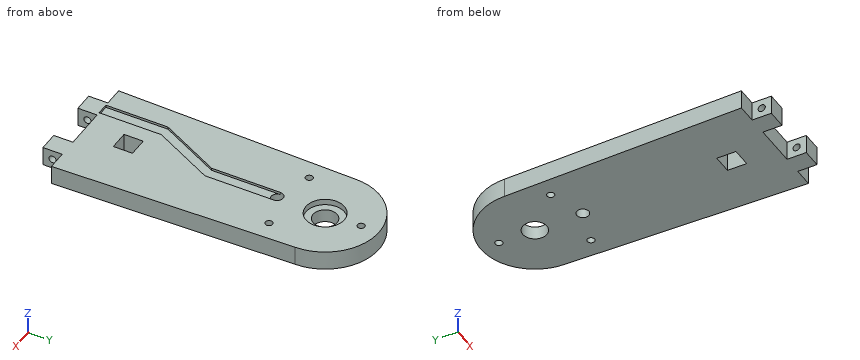
```python
from build123d import *

# Parameters (mm, degrees)
ARM_BOSS_EXTRUDE1_DEPTH                    = 8
SKETCH2_R                                  = 8
BEARING_CUT_EXTRUDE1_DEPTH                 = 2.5
SKETCH3_R                                  = 5
SHAFT_HOLE_CUT_EXTRUDE2_DEPTH              = 5.5
SKETCH4_R                                  = 2.5
CABLE_HOLE_CUT_EXTRUDE3_DEPTH              = 8
SKETCH5_W                                  = 8
SKETCH5_H                                  = 8
PUZZLE_SLOT_BOSS_EXTRUDE2_DEPTH            = 8
SKETCH6_W                                  = 5
SKETCH6_H                                  = 7.5
CABLE_CUT_EXTRUDE4_DEPTH                   = 1
SKETCH7_R                                  = 1.5
MOUNTING_HOLES_CUT_EXTRUDE5_DEPTH          = 8
PUZZLE_SLOT_SCREW_HOLES_CUT_EXTRUDE6_REACH = 118.155
SKETCH8_R                                  = 1.5
SIDE_PUZZLE_SLOT_CUT_EXTRUDE7_DEPTH        = 8
CABLE_LOWER_CUT_EXTRUDE8_DEPTH             = 1


with BuildPart() as part:
    # Sketch1 → Arm Boss-Extrude1 (new body)
    with BuildSketch(Plane.XY):
        with BuildLine():
            Line((-22.5, 0), (-25, -100))
            Line((-25, -100), (0, -100))
            Line((0, -100), (25, -100))
            Line((25, -100), (22.5, 0))
            ThreePointArc((22.5, 0), (0, 22.5), (-22.5, 0))
        make_face()
    extrude(amount=-ARM_BOSS_EXTRUDE1_DEPTH)

    # Sketch2 → Bearing Cut-Extrude1 (cut)
    with BuildSketch(Plane.XY):
        Circle(SKETCH2_R)
    extrude(amount=-BEARING_CUT_EXTRUDE1_DEPTH, mode=Mode.SUBTRACT)

    # Sketch3 → Shaft Hole Cut-Extrude2 (cut)
    with BuildSketch(Plane.XY.offset(-2.5)):
        Circle(SKETCH3_R)
    extrude(amount=-SHAFT_HOLE_CUT_EXTRUDE2_DEPTH, mode=Mode.SUBTRACT)

    # Sketch4 → Cable Hole Cut-Extrude3 (cut)
    with BuildSketch(Plane.XY):
        with Locations((0, -20)):
            Circle(SKETCH4_R)
    extrude(amount=-CABLE_HOLE_CUT_EXTRUDE3_DEPTH, mode=Mode.SUBTRACT)

    # Sketch5 → Puzzle Slot Boss-Extrude2 (add)
    with BuildSketch(Plane.XZ.offset(100)):
        with Locations((-13, -4)):
            Rectangle(SKETCH5_W, SKETCH5_H)
        with Locations((13, -4)):
            Rectangle(SKETCH5_W, SKETCH5_H)
    extrude(amount=PUZZLE_SLOT_BOSS_EXTRUDE2_DEPTH)

    # Sketch6 → Cable Cut-Extrude4 (cut)
    with BuildSketch(Plane.XY):
        with Locations((0, -23.75)):
            Rectangle(SKETCH6_W, SKETCH6_H)
    extrude(amount=-CABLE_CUT_EXTRUDE4_DEPTH, mode=Mode.SUBTRACT)

    # Sketch7 → Mounting Holes Cut-Extrude5 (cut)
    with BuildSketch(Plane.XY):
        with Locations((-15, -15)):
            Circle(SKETCH7_R)
        with Locations((15, -15)):
            Circle(SKETCH7_R)
        with Locations((0, 15)):
            Circle(SKETCH7_R)
    extrude(amount=-MOUNTING_HOLES_CUT_EXTRUDE5_DEPTH, mode=Mode.SUBTRACT)

    # Puzzle Slot Screw Holes Cut-Extrude6: up to this face of the body (flat: up to its plane)
    puzzle_slot_screw_holes_cut_extrude6_end = Plane(part.part.faces().sort_by_distance((17, -104, -4))[0])
    # Sketch8 → Puzzle Slot Screw Holes Cut-Extrude6 (cut, up to the picked face)
    with BuildSketch(Plane.ZY.offset(17), mode=Mode.PRIVATE) as puzzle_slot_screw_holes_cut_extrude6_sk1:
        with Locations((-4, -104)):
            Circle(SKETCH8_R)
    puzzle_slot_screw_holes_cut_extrude6_tool1 = split(extrude(puzzle_slot_screw_holes_cut_extrude6_sk1.sketch, amount=-PUZZLE_SLOT_SCREW_HOLES_CUT_EXTRUDE6_REACH, mode=Mode.PRIVATE), bisect_by=puzzle_slot_screw_holes_cut_extrude6_end, keep=Keep.BOTH, mode=Mode.PRIVATE)
    add(puzzle_slot_screw_holes_cut_extrude6_tool1.solids().sort_by(Axis((-17, -104, -4), (1, 0, 0)))[0], mode=Mode.SUBTRACT)

    # Sketch9 → Side Puzzle Slot Cut-Extrude7 (cut)
    with BuildSketch(Plane.XY):
        Polygon((-4, -78), (0, -78), (4, -78), (4, -86), (-4, -86), align=None)
    extrude(amount=-SIDE_PUZZLE_SLOT_CUT_EXTRUDE7_DEPTH, mode=Mode.SUBTRACT)

    # Sketch10 → Cable Lower Cut-Extrude8 (cut)
    with BuildSketch(Plane.XY):
        Polygon((-15.5, -100), (-10.5, -100), (-10.5, -74.117724453), (2.5, -48.683858805), (2.5, -27.5), (-2.5, -27.5), (-2.5, -48.683858805), (-15.5, -74.117724453), align=None)
    extrude(amount=-CABLE_LOWER_CUT_EXTRUDE8_DEPTH, mode=Mode.SUBTRACT)


solid = part.part
```
Input: part model. Units: mm. Frame: model coordinates. Give positions to 0.01 mm unless a question says otherwise; leave off trailing zeros. Order: outer loops, then holes, each group sorted by start corner. A loop starts at its lowest first (then second) coordinate and runs counter-clockwise, first axis right, second up. Notation, with made-up numbers: (63.5, 63) - (81.5, 63) arc R20 ccw to (81.5, 101) - close; hole circle Ø4 at (-9, 56.25). An arc over 180 degrees is marked (long way). Use a Markdown table: item, result.
(1) Pin query (flat end, axial travel): pin 1 (1.5 mm diameter, centred on y = -3.5, z = -2.5, fed in from +X); pin 2 (4 mm diameter, centred on x = 16.5, y = -11, fed in from +Z); pin 3 (2 mm diameter, centred on x = 11.5, z = -2, fed in from +Y); pin 4 (1.8 mm diameter, centred on y = -104, z = -4, fed in from +X). Return the tip coordinate at first contact, or that it passes through.
Computed values:
| item | result |
|---|---|
| pin 1 | stops at x = 22.61 |
| pin 2 | stops at z = 0 |
| pin 3 | stops at y = 19.9 |
| pin 4 | passes through |
(2) Line query: line 1 (Y direction, x = 0, z = -5.5); line 2 (Y direction, x = 0, z = -1.25); line 3 (Z direction, x = 15.25, y = -104). Output: solid intervals per line, ascending. Write a range as from..to.
Computed values:
| item | result |
|---|---|
| line 1 | y = -100..-86, -78..-22.5, -17.5..-5, 5..13.5, 16.5..22.5 |
| line 2 | y = -100..-86, -78..-22.5, -17.5..-8, 8..13.5, 16.5..22.5 |
| line 3 | z = -8..-5.5, -2.5..0 |
(3) Section query A-A (z = -4). State how many separate pieces and enclosed holes the cut face has, then the cut area to 3 significant figures.
Computed values:
| item | result |
|---|---|
| separate pieces | 3 |
| enclosed holes | 6 |
| area | 5,440 mm2 |
(4) Section query B-B (y = -104). Output: boundary loops of the cut face in (x, z).
Computed values:
| item | result |
|---|---|
| outline | (-17, -8) - (-9, -8) - (-9, -5.5) - (-17, -5.5) - close; (-17, -2.5) - (-9, -2.5) - (-9, 0) - (-17, 0) - close; (9, -8) - (17, -8) - (17, -5.5) - (9, -5.5) - close; (9, -2.5) - (17, -2.5) - (17, 0) - (9, 0) - close |
(5) Section query C-C (x = 15). Output: boundary loops of the cut face in (y, z).
Computed values:
| item | result |
|---|---|
| outline | (-108, -8) - (-16.5, -8) - (-16.5, 0) - (-108, 0) - close; (-13.5, -8) - (16.77, -8) - (16.77, 0) - (-13.5, 0) - close; hole circle Ø3 at (-104, -4) |
(6) Section query D-D (y = -90). Output: boundary loops of the cut face in (x, z).
Computed values:
| item | result |
|---|---|
| outline | (-24.75, -8) - (24.75, -8) - (24.75, 0) - (-10.5, 0) - (-10.5, -1) - (-15.5, -1) - (-15.5, 0) - (-24.75, 0) - close |
